Source: CAD feature listing. Evaluate the final solid. Frame: model axes, mm. A direction names the side the tool comes from. Coordinates: 2 decimals unless noted, no trailing zeros. Loops run counter-clockwise (first coordinate to the right, second up) from the corner with the lowest first, then second, coordinate; pieces in that order, holes last.
Item 1: Section query B-B, the plane y = -4.6. Return the cut outline in (x, z).
Item 2: Pin query (flat end, axial travel): pin 1 Ø3 at (x, y) = (121.2, -17.13) entering from -Z; pin 2 Ø1.5 at (x, y) = (20, -8.5) entering from -Z; pin 3 Ø2 at (x, z) = (4.5, 2.5) entering from -Y. Return the tip coordinate at first contact, or that it passes through.
Item 3: Pull-direction query (X, two-part tool) for faces 4 (the flat face through (-30.2, 0, 2)), 5 (the cylindrical face through (78.21, 2.75, 1.97)), 6 (the flat face through (0, -10.1, 2)), 7 (the flat face through (32, -1, 4)); classes: +X half, -X half, draft (parallel to the pull), parting line (faces both ways), or undercut.
Item 4: Line query: probe 1 along Y at (x, z) = (-25.2, 0.95); probe 2 along Y at (x, z) = (8, 3.75); probe 3 along X at (y, z) = (-16, 3.7). Output: solid intervals per line, ascending.
Item 5: Section query C-C, the plane x = 121.2. Return the cut outline in (y, z), then the cut area to 3 significant figures.
Item 6: Section query D-D, the plane z = 0.65. Return the cut outline in (x, y).
Item 7: Reachability of faces 1 (the flat face through (-5, -17.1, 2)), 2 (the flat face through (0, 10.1, 2)), 3 (the flat face through (32, -1, 0)) from +Z, -Z, +X, -X, +Y, -Y: full face, straight path, thin tool, end or side. Return the list, or none.
Item 8: Section query A-A, the plane x = -25.2. Return the cut outline in (y, z), then the cut area to 3 significant figures.
```python
from build123d import *

# Parameters (mm, degrees)
SZKIC2_R                    = 2.35
SZKIC2_R_2                  = 1.75
SZKIC2_W                    = 40.4
SZKIC2_H                    = 20.2
DODANIE_WYCI_GNI_CIE1_DEPTH = 4


with BuildPart() as part:
    # Szkic2 → Dodanie-wyciągnięcie1 (new body)
    with BuildSketch(Plane.XY):
        with BuildLine():
            Line((-30.2, 17.1), (30.2, 17.1))
            ThreePointArc((30.2, 17.1), (78.887653554, 2.515256091), (126.216652739, -16.009543491))
            ThreePointArc((126.216652739, -16.009543491), (127.600370297, -18.154974458), (126.269263581, -20.333437957))
            ThreePointArc((126.269263581, -20.333437957), (72.757727431, -17.908543704), (19.197379501, -17.1))
            Line((19.197379501, -17.1), (-30.2, -17.1))
            Line((-30.2, -17.1), (-30.2, 17.1))
        make_face()
        with Locations((-25.2, 4.6)):
            Circle(SZKIC2_R, mode=Mode.SUBTRACT)
        with Locations(Location((25.2, 4.6, 0), (0, 0, 180))):
            Circle(SZKIC2_R, mode=Mode.SUBTRACT)
        with Locations((25.2, -4.6)):
            Circle(SZKIC2_R, mode=Mode.SUBTRACT)
        with Locations(Location((-25.2, -4.6, 0), (0, 0, 180))):
            Circle(SZKIC2_R, mode=Mode.SUBTRACT)
        with Locations((121.2, -17.133437957)):
            Circle(SZKIC2_R_2, mode=Mode.SUBTRACT)
        Rectangle(SZKIC2_W, SZKIC2_H, mode=Mode.SUBTRACT)
    extrude(amount=DODANIE_WYCI_GNI_CIE1_DEPTH)


solid = part.part
```
Verdict:
1. outline: (-30.2, 0) - (-27.55, 0) - (-27.55, 4) - (-30.2, 4) - close; (-22.85, 0) - (-20.2, 0) - (-20.2, 4) - (-22.85, 4) - close; (20.2, 0) - (22.85, 0) - (22.85, 4) - (20.2, 4) - close; (27.55, 0) - (98.45, 0) - (98.45, 4) - (27.55, 4) - close
2. pin 1: passes through
2. pin 2: stops at z = 0
2. pin 3: stops at y = -17.1
3. face 4: -X half
3. face 5: +X half
3. face 6: undercut
3. face 7: draft
4. probe 1: y = -17.1 to -6.95, -2.25 to 2.25, 6.95 to 17.1
4. probe 2: y = -17.1 to -10.1, 10.1 to 17.1
4. probe 3: x = -30.2 to 119.87, 122.53 to 126.19
5. outline: (-20.03, 0) - (-18.88, 0) - (-18.88, 4) - (-20.03, 4) - close; (-15.38, 0) - (-13.83, 0) - (-13.83, 4) - (-15.38, 4) - close
5. area: 10.8 mm2
6. outline: (-30.2, -17.1) - (19.2, -17.1) arc R1774.4 cw to (126.27, -20.33) arc R2.4 ccw to (126.22, -16.01) arc R619.81 ccw to (30.2, 17.1) - (-30.2, 17.1) - close; hole circle Ø4.7 at (-25.2, -4.6); hole circle Ø4.7 at (-25.2, 4.6); hole (-20.2, -10.1) - (20.2, -10.1) - (20.2, 10.1) - (-20.2, 10.1) - close; hole circle Ø4.7 at (25.2, -4.6); hole circle Ø4.7 at (25.2, 4.6); hole circle Ø3.5 at (121.2, -17.13)
7. face 1: +Z, -Z, -X, -Y
7. face 2: +Z, -Z
7. face 3: -Z, +X, -X, +Y, -Y
8. outline: (-17.1, 0) - (-6.95, 0) - (-6.95, 4) - (-17.1, 4) - close; (-2.25, 0) - (2.25, 0) - (2.25, 4) - (-2.25, 4) - close; (6.95, 0) - (17.1, 0) - (17.1, 4) - (6.95, 4) - close
8. area: 99.2 mm2
